```python
from build123d import *

# Parameters (mm, degrees)
SKETCH1_W            = 1150
SKETCH1_H            = 35
BOSS_EXTRUDE1_DEPTH  = 28
SKETCH4_W            = 38.3
SKETCH4_H            = 35
BOSS_EXTRUDE4_DEPTH  = 307.4
BOSS_EXTRUDE5_DEPTH  = 38.3
BOSS_EXTRUDE6_DEPTH  = 38.3
SKETCH7_W            = 38.3
SKETCH7_H            = 39.4
BOSS_EXTRUDE7_DEPTH  = 38.5
SKETCH8_W            = 39.4
SKETCH8_H            = 38.5
BOSS_EXTRUDE8_DEPTH  = 901.7
SKETCH9_W            = 38.3
SKETCH9_H            = 38.5
BOSS_EXTRUDE9_DEPTH  = 90
SKETCH11_W           = 6
SKETCH11_H           = 56
BOSS_EXTRUDE10_DEPTH = 77
FILLET1_R            = 10
CUT_EXTRUDE1_REACH   = 1252.131
SKETCH12_R           = 6.3
SHELL1_START         = -467
SHELL1_OUTLINE_W     = 32.5
SHELL1_OUTLINE_H     = 33.4
SHELL1_OUTLINE_W_2   = 29
SHELL1_OUTLINE_H_2   = 50
SHELL1_DEPTH         = 934
SHELL1_2_DEPTH       = 32.3
SHELL1_START_2       = 434.7
SHELL1_3_DEPTH       = 32.3
SHELL1_START_3       = -572
SHELL1_4_OUTLINE_W   = 29
SHELL1_4_OUTLINE_H   = 50
SHELL1_4_DEPTH       = 1147
BOSS_EXTRUDE12_REACH = 830.567
SKETCH17_W           = 3
SKETCH17_H           = 50
FILLET2_R            = 2
CUT_EXTRUDE2_START   = -940
SKETCH18_R           = 10
CUT_EXTRUDE2_DEPTH   = 940


# Read off the part's stored shape, not the designer's step: Shell1
with BuildPart() as part:
    # Sketch1 → Boss-Extrude1 (new, symmetric)
    with BuildSketch(Plane.XY):
        Rectangle(SKETCH1_W, SKETCH1_H)
    extrude(amount=BOSS_EXTRUDE1_DEPTH, both=True)

    # Sketch4 → Boss-Extrude4 (add)
    with BuildSketch(Plane(origin=(0, 0, -28), x_dir=(-1, 0, 0), z_dir=(0, 0, -1))):
        with Locations((-450.85, 0)):
            Rectangle(SKETCH4_W, SKETCH4_H)
        with Locations((450.85, 0)):
            Rectangle(SKETCH4_W, SKETCH4_H)
    extrude(amount=BOSS_EXTRUDE4_DEPTH)

    # Sketch5 → Boss-Extrude5 (add)
    with BuildSketch(Plane(origin=(470, 0, 0), x_dir=(0, 0, -1), z_dir=(1, 0, 0))):
        Polygon((335.4, -17.5), (296, -17.5), (142.090935503, -440.361679354), (181.490935503, -440.361679354), align=None)
    extrude(amount=-BOSS_EXTRUDE5_DEPTH)

    # Sketch6 → Boss-Extrude6 (add)
    with BuildSketch(Plane(origin=(-431.7, 0, 0), x_dir=(0, 0, -1), z_dir=(1, 0, 0))):
        Polygon((335.4, -17.5), (296, -17.5), (142.090935503, -440.361679354), (181.490935503, -440.361679354), align=None)
    extrude(amount=-BOSS_EXTRUDE6_DEPTH)

    # Sketch7 → Boss-Extrude7 (add)
    with BuildSketch(Plane.XZ.offset(440.361679354)):
        with Locations((450.85, -161.790935503)):
            Rectangle(SKETCH7_W, SKETCH7_H)
    extrude(amount=BOSS_EXTRUDE7_DEPTH)

    # Sketch8 → Boss-Extrude8 (add)
    with BuildSketch(Plane.ZY.offset(-431.7)):
        with Locations((-161.790935503, -459.611679354)):
            Rectangle(SKETCH8_W, SKETCH8_H)
    extrude(amount=BOSS_EXTRUDE8_DEPTH)

    # Sketch9 → Boss-Extrude9 (add)
    with BuildSketch(Plane.XY.offset(-142.090935503)):
        with Locations((-450.85, -459.611679354)):
            Rectangle(SKETCH9_W, SKETCH9_H)
        with Locations((450.85, -459.611679354)):
            Rectangle(SKETCH9_W, SKETCH9_H)
    extrude(amount=BOSS_EXTRUDE9_DEPTH)

    # Sketch11 → Boss-Extrude10 (add)
    with BuildSketch(Plane.XZ.offset(17.5)):
        with Locations((-527, 0)):
            Rectangle(SKETCH11_W, SKETCH11_H)
        with Locations((-306, 0)):
            Rectangle(SKETCH11_W, SKETCH11_H)
        with Locations((317, 0)):
            Rectangle(SKETCH11_W, SKETCH11_H)
        with Locations((534, 0)):
            Rectangle(SKETCH11_W, SKETCH11_H)
    extrude(amount=BOSS_EXTRUDE10_DEPTH)

    # Fillet1
    fillet1_edges = [part.edges().sort_by_distance(p)[0] for p in [
        (-527, -94.5, 28),
        (-527, -94.5, -28),
        (-306, -94.5, 28),
        (-306, -94.5, -28),
        (534, -94.5, 28),
        (534, -94.5, -28),
        (317, -94.5, 28),
        (317, -94.5, -28),
    ]]
    fillet(fillet1_edges, radius=FILLET1_R)

    # Cut-Extrude1: up to this face of the body (flat: up to its plane)
    cut_extrude1_end = Plane(part.part.faces().sort_by_distance((537, -55.635386562, 0))[0])
    # Sketch12 → Cut-Extrude1 (cut, up to the picked face)
    with BuildSketch(Plane.ZY.offset(530), mode=Mode.PRIVATE) as cut_extrude1_sk1:
        with Locations(Location((0, -81.3, 0), (0, 0, 180))):
            Circle(SKETCH12_R)
    cut_extrude1_tool1 = split(extrude(cut_extrude1_sk1.sketch, amount=-CUT_EXTRUDE1_REACH, mode=Mode.PRIVATE), bisect_by=cut_extrude1_end, keep=Keep.BOTH, mode=Mode.PRIVATE)
    add(cut_extrude1_tool1.solids().sort_by(Axis((-530, -81.3, 0), (1, 0, 0)))[0], mode=Mode.SUBTRACT)

    # Shell1 outline → Shell1 (cut)
    with BuildSketch(Plane.YZ.offset(SHELL1_START)):
        with Locations((-459.611679354, -161.790935503)):
            Rectangle(SHELL1_OUTLINE_W, SHELL1_OUTLINE_H)
        Rectangle(SHELL1_OUTLINE_W_2, SHELL1_OUTLINE_H_2)
    extrude(amount=SHELL1_DEPTH, mode=Mode.SUBTRACT)

    # Shell1 2 outline → Shell1 2 (cut)
    with BuildSketch(Plane.YZ.offset(SHELL1_START)):
        Polygon((-475.861679354, -55.090935503), (-475.861679354, -145.090935503), (-443.361679354, -145.090935503), (-443.361679354, -178.490935503), (-439.832698412, -178.490935503), (-16.971019058, -332.4), (14.5, -332.4), (14.5, -25), (-14.5, -25), (-14.5, -300.28444402), (-443.361679354, -144.191558118), (-443.361679354, -55.090935503), align=None)
    extrude(amount=SHELL1_2_DEPTH, mode=Mode.SUBTRACT)

    # Shell1 3 outline → Shell1 3 (cut)
    with BuildSketch(Plane.YZ.offset(SHELL1_START_2)):
        Polygon((-475.861679354, -55.090935503), (-475.861679354, -145.090935503), (-443.361679354, -145.090935503), (-443.361679354, -178.490935503), (-439.832698412, -178.490935503), (-16.971019058, -332.4), (14.5, -332.4), (14.5, -25), (-14.5, -25), (-14.5, -300.28444402), (-443.361679354, -144.191558118), (-443.361679354, -55.090935503), align=None)
    extrude(amount=SHELL1_3_DEPTH, mode=Mode.SUBTRACT)

    # Shell1 4 outline → Shell1 4 (cut)
    with BuildSketch(Plane.YZ.offset(SHELL1_START_3)):
        Rectangle(SHELL1_4_OUTLINE_W, SHELL1_4_OUTLINE_H)
    extrude(amount=SHELL1_4_DEPTH, mode=Mode.SUBTRACT)

    # Sketch17 → Boss-Extrude12 (add, up to next)
    with BuildSketch(Plane.XZ.offset(-14.5), mode=Mode.PRIVATE) as boss_extrude12_sk1:
        with Locations((573.5, 0)):
            Rectangle(SKETCH17_W, SKETCH17_H)
    boss_extrude12_tool1 = extrude(boss_extrude12_sk1.sketch, amount=BOSS_EXTRUDE12_REACH, mode=Mode.PRIVATE) - part.part
    add(boss_extrude12_tool1.solids().sort_by_distance((573.5, 14.5, 0))[0])

    # Fillet2
    fillet2_edges = [part.edges().sort_by_distance(p)[0] for p in [
        (-530, -17.5, 0),
        (-524, -17.5, 0),
        (-309, -17.5, 0),
        (-303, -17.5, 0),
        (531, -17.5, 0),
        (537, -17.5, 0),
        (314, -17.5, 0),
        (320, -17.5, 0),
    ]]
    fillet(fillet2_edges, radius=FILLET2_R)

    # Sketch18 → Cut-Extrude2 (cut)
    with BuildSketch(Plane(origin=(470, 0, 0), x_dir=(0, 0, -1), z_dir=(1, 0, 0)).offset(CUT_EXTRUDE2_START)):
        with Locations((82.090935503, -459.611679354)):
            Circle(SKETCH18_R)
    extrude(amount=CUT_EXTRUDE2_DEPTH, mode=Mode.SUBTRACT)


solid = part.part
```
Check sheet for the modelled part. Datum: model origin and axes. Units: mm. A direction names the side the tool comes from. Coordinates: 2 decimals unless noted, no trailing zeros. Loops run counter-clockwise (first coordinate to the right, second up) from the corner with the lowest first, then second, coordinate; pieces in that order, holes last.
1) Material ranges on probe 1 along Y at (x, z) = (-526, 0); probe 2 along Y at (x, z) = (180.5, -1.5); probe 3 along Z at (x, y) = (-304, -81), recorded low to high.
2) Sectioned sample at A-A (x = -41). Record the boundary of the cut face in (y, z), and give its area (3 significant figures).
3) Access from +Z, -Z, +X, -X, +Y, -Y to the whole of each face (thin tool, end or side, straight path). Record for faces 1 (the face through (1, -17.5, 0)), 2 (the face through (-520, 0, -25)), 3 (the face through (470, -174.4, -239.3)), 4 (the face through (6, -460, -142.091)), 5 (the face through (-450.582, -225.971, -220.123)).
4) Sectioned sample at B-B (y = -64). Count the separate pieces of the cut face and the enclosed holes in it, and give its area (3 significant figures).
5) Release check for a two-part mould opening along Z. For faces 6 (the face through (-6, 0, -25)), 7 (the face through (-470, -213, -239)), 8 (the face through (-523, 1, -28)) record: released by +Z, released by -Z, zero draft, split by the parting line, or undercut.
6) Gauge pin test, flat ends, axial feed: pin 1 (16 mm diameter, centred on x = -452, y = -462, fed in from -Z); pin 2 (11.5 mm diameter, centred on x = -453, y = -462, fed in from +Z); pin 3 (17 mm diameter, centred on y = -63.5, z = 13.5, fed in from -X). Record the tip position at first contact, or that the pin passes through.
Check sheet entries:
1. probe 1: y = -94.5 to -87.6, -75 to -14.5, 14.5 to 17.5
1. probe 2: y = -17.5 to -14.5, 14.5 to 17.5
1. probe 3: z = -28 to -6.29, 6.29 to 28
2. outline: (-478.86, -181.49) - (-440.36, -181.49) - (-440.36, -142.09) - (-478.86, -142.09) - close; (-17.5, -28) - (17.5, -28) - (17.5, 28) - (-17.5, 28) - close; hole (-475.86, -178.49) - (-443.36, -178.49) - (-443.36, -145.09) - (-475.86, -145.09) - close; hole (-14.5, -25) - (14.5, -25) - (14.5, 25) - (-14.5, 25) - close
2. area: 941 mm2
3. face 1: +Z, -Z, -Y
3. face 2: none
3. face 3: -Z, +X, +Y, -Y
3. face 4: +Z, +Y, -Y
3. face 5: +Z, +X, -X
4. separate pieces: 6
4. enclosed holes: 2
4. area: 2,230 mm2
5. face 6: undercut
5. face 7: zero draft
5. face 8: released by -Z
6. pin 1: stops at z = -181.49
6. pin 2: stops at z = -52.09
6. pin 3: stops at x = -530
